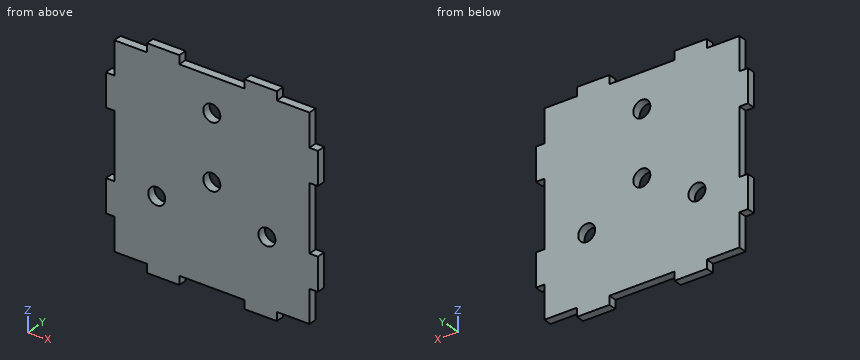
from build123d import *

# Parameters (mm, degrees)
BOSS_EXTRUDE1_DEPTH = 6
SKETCH2_R           = 6
CUT_EXTRUDE1_DEPTH  = 107.235587258
CIRPATTERN1_COUNT   = 3


with BuildPart() as part:
    # Sketch1 → Boss-Extrude1 (new body)
    with BuildSketch(Plane(origin=(0, 0, 0), x_dir=(1, 0, 0), z_dir=(0, 1, 0))):
        Polygon((0, 69), (-23, 69), (-23, 75), (-46, 75), (-46, 69), (-69, 69), (-69, 46), (-75, 46), (-75, 23), (-69, 23), (-69, 0), (-69, -23), (-75, -23), (-75, -46), (-69, -46), (-69, -69), (-46, -69), (-46, -75), (-23, -75), (-23, -69), (0, -69), (23, -69), (23, -75), (46, -75), (46, -69), (69, -69), (69, -46), (75, -46), (75, -23), (69, -23), (69, 0), (69, 23), (75, 23), (75, 46), (69, 46), (69, 69), (46, 69), (46, 75), (23, 75), (23, 69), align=None)
    extrude(amount=BOSS_EXTRUDE1_DEPTH)

    # Sketch2 → Cut-Extrude1 (cut, through all)
    with BuildSketch(Plane(origin=(0, 6, 0), x_dir=(1, 0, 0), z_dir=(0, 1, 0))):
        with Locations(Location((0, 0, 0), (0, 0, 270))):
            Circle(SKETCH2_R)
        with Locations(Location((0, -45, 0), (0, 0, 270))):
            Circle(SKETCH2_R)
    cut_extrude1 = extrude(amount=-CUT_EXTRUDE1_DEPTH, mode=Mode.SUBTRACT)

    # CirPattern1: Cut-Extrude1 ×3 about axis
    cirpattern1_axis = Axis((0, 0, 0), (0, 1, 0))
    for i in range(1, CIRPATTERN1_COUNT):
        add(cut_extrude1.rotate(cirpattern1_axis, i * 360 / CIRPATTERN1_COUNT), mode=Mode.SUBTRACT)


solid = part.part
Work out the finished part from the listing and answer in its coordinate system (mm). Coordinates: 2 decimals unless noted, no trailing zeros. Order: outer loops, then holes, each group sorted by start corner. A loop starts at its lowest first (then second) coordinate and runs counter-clockwise, first axis right, second up. Notation, with made-up numbers: (77.5, -13) - (123.5, -13) arc R17 ccw to (123.5, 7) - close; hole circle Ø6 at (2, 7). An arc over 180 degrees is marked (long way). Put each result on its own line as item: value. Start each with the question number.
1) Find section B-B (z = 0). Give the vertices of the cut face in (x, y), plus the area to 3 significant figures.
2) Find section D-D (y = 2.7). State how many separate pieces and enclosed holes the cut face has, plus the area to 3 significant figures.
3) Find section A-A (x = 0). Give the vertices of the cut face in (y, z), plus the area to 3 significant figures.
4) Flat-ended cylindrical pins translate along their axes: pin 1 (1.8 mm diameter, centred on x = -72, y = 2.5, fed in from -Z); pin 2 (1.8 mm diameter, centred on y = 3.5, z = -10.5, fed in from -X); pin 3 (3 mm diameter, centred on y = 2, z = 71, fed in from +X). Find the tip coordinate at first contact, or state that the pin passes through.
5) Find section C-C (x = -36). Give the vertices of the cut face in (y, z).
6) Find the intervals of material crossed by line 1 (X direction, y = 4.35, z = -22.5); line 2 (X direction, y = 1.7, z = 0); line 3 (Z direction, x = 66.5, y = 1.1), in increasing order. Write a range as from..to.
Results list:
1. outline: (-69, 0) - (-6, 0) - (-6, 6) - (-69, 6) - close; (6, 0) - (69, 0) - (69, 6) - (6, 6) - close
1. area: 756 mm^2
2. separate pieces: 1
2. enclosed holes: 4
2. area: 19,700 mm^2
3. outline: (0, -69) - (6, -69) - (6, -6) - (0, -6) - close; (0, 6) - (6, 6) - (6, 39) - (0, 39) - close; (0, 51) - (6, 51) - (6, 69) - (0, 69) - close
3. area: 684 mm^2
4. pin 1: stops at z = -46
4. pin 2: stops at x = -69
4. pin 3: stops at x = 46
5. outline: (0, -75) - (6, -75) - (6, -27.71) - (0, -27.71) - close; (0, -17.29) - (6, -17.29) - (6, 75) - (0, 75) - close
6. line 1: x = -69..-44.97, -32.97..32.97, 44.97..69
6. line 2: x = -69..-6, 6..69
6. line 3: z = -69..69
